Here's how the part is built. I have some questions about the finished solid (model axes, mm). A direction names the side the tool comes from. Give positions to 0.01 mm unless a question says otherwise; leave off trailing zeros. Loops run counter-clockwise (first coordinate to the right, second up) from the corner with the lowest first, then second, coordinate; pieces in that order, holes last.
Q1. I need wall thicknesses on line 1 (Z direction, x = -4, y = -133.5); line 2 (Y direction, x = -10.5, z = 16); line 3 (Y direction, x = 19, z = -8). Which ranges of each line are inside material? Lowest first, please.
Q2. If we section it at C-C (x = -30): Please give me the cut outline in (y, z).
Q3. We'd pull the mould along Y, two halves only. Please class faces 1 (the face through (16.298, -31.804, 2.099)), 2 (the face through (30.935, -58, 1)), 3 (the face through (-8, 0, 2)): +Y half, -Y half, draft (parallel to the pull), parting line (faces both ways), or undercut.
Q4. For faces 4 (the face through (-7, -101.589, 20)), 5 (the face through (-8, -152.4, -17)), which set-ups out of +Z, -Z, +X, -X, +Y, -Y let a thin tool reach every point of the face, with its end or its side?
Q5. If we section it at A-A (x = -5): Please give me the cut outline in (y, z).
Q6. If we section it at B-B (y = -138.5): Please give me the cut outline in (x, z), plus the area to 3 significant figures.
Q7. If we section it at D-D (z = 20.5): Please give me the cut outline in (x, y).
Q8. Will this pin go through, and if not, where does the flat tip stop? P1, Ø15, axis at x = 6.5, y = -125, coming from the +Z side.
from build123d import *

# Parameters (mm, degrees)
F0_W     = 76.189154759
F0_H     = 76.2136504054
F1_DEPTH = 152.4
F2_W     = 50.8111025929
F2_H     = 38.1068252027
F3_DEPTH = 76.2
F4_R     = 6.3508418906
F4_R_2   = 6.3510810939
F5_DEPTH = 101.6


with BuildPart() as f1:
    # F0 (on Front) → F1 (new body)
    with BuildSketch(Plane.XZ):
        with Locations((-7.1593066677, 1.5659481287)):
            Rectangle(F0_W, F0_H)
    extrude(amount=F1_DEPTH)

    # F2 (on face) → F3 (cut)
    with BuildSketch(Plane.YZ.offset(30.9352707118)):
        with Locations((-126.9944487035, 20.6193607301)):
            Rectangle(F2_W, F2_H)
    extrude(amount=-F3_DEPTH, mode=Mode.SUBTRACT)

    # F4 (on face) → F5 (cut)
    with BuildSketch(Plane.XY.offset(39.6727733314)):
        with Locations((-30.4293371737, -38.1011925638)):
            Circle(F4_R)
        with Locations((17.1245448291, -38.1011925638)):
            Circle(F4_R_2)
    extrude(amount=-F5_DEPTH, mode=Mode.SUBTRACT)


solid = f1.part
Check sheet entries:
1. line 1: z = -36.54 to 1.57
1. line 2: y = -101.59 to 0
1. line 3: y = -152.4 to -44.17, -32.03 to 0
2. outline: (-152.4, -36.54) - (-44.44, -36.54) - (-44.44, 39.67) - (-101.59, 39.67) - (-101.59, 1.57) - (-152.4, 1.57) - close; (-31.76, -36.54) - (0, -36.54) - (0, 39.67) - (-31.76, 39.67) - close
3. face 1: undercut
3. face 2: draft
3. face 3: +Y half
4. face 4: +Z, +X, -X, -Y
4. face 5: +Z, -Z, +X, -X, -Y
5. outline: (-152.4, -36.54) - (0, -36.54) - (0, 39.67) - (-101.59, 39.67) - (-101.59, 1.57) - (-152.4, 1.57) - close
6. outline: (-45.25, -36.54) - (30.94, -36.54) - (30.94, 1.57) - (-45.25, 1.57) - close
6. area: 2,900 mm2
7. outline: (-45.25, -101.59) - (30.94, -101.59) - (30.94, 0) - (-45.25, 0) - close; hole circle Ø12.7 at (-30.43, -38.1); hole circle Ø12.7 at (17.12, -38.1)
8. P1: stops at z = 1.57
